from build123d import *

# Parameters (mm, degrees)
SKETCH_R        = 35
PAD_DEPTH       = 7
SKETCH002_R     = 11
POCKET_DEPTH    = 7
SKETCH003_R     = 5.25
POCKET001_DEPTH = 4
SKETCH004_R     = 2.625
POCKET002_DEPTH = 1


with BuildPart() as part:
    # Sketch → Pad (new body)
    with BuildSketch(Plane.XY):
        Circle(SKETCH_R)
    extrude(amount=PAD_DEPTH)

    # Sketch002 → Pocket (cut)
    with BuildSketch(Plane(origin=(0, 0, 0), x_dir=(1, 0, 0), z_dir=(0, 0, -1))):
        Circle(SKETCH002_R)
    extrude(amount=-POCKET_DEPTH, mode=Mode.SUBTRACT)

    # Sketch003 (on Face3 of Pocket) → Pocket001 (cut)
    with BuildSketch(Plane.XY.offset(7)):
        with Locations((20, 0)):
            Circle(SKETCH003_R)
        with Locations((-20, 0)):
            Circle(SKETCH003_R)
    extrude(amount=-POCKET001_DEPTH, mode=Mode.SUBTRACT)

    # Sketch004 (on Face7 of Pocket001) → Pocket002 (cut)
    with BuildSketch(Plane.XY.offset(3)):
        with Locations((-20, 0)):
            Circle(SKETCH004_R)
        with Locations((20, 0)):
            Circle(SKETCH004_R)
    extrude(amount=-POCKET002_DEPTH, mode=Mode.SUBTRACT)


solid = part.part
The model under review builds one solid part; all positions refer to its coordinate system, in mm. A direction names the side the tool comes from. Give positions to 0.01 mm unless a question says otherwise; leave off trailing zeros. Loops run counter-clockwise (first coordinate to the right, second up) from the corner with the lowest first, then second, coordinate; pieces in that order, holes last. Notation, with made-up numbers: (57.5, 20.5) -> (86.5, 20.5) arc R15 ccw to (86.5, 49.5) -> close; hole circle Ø11 at (-0.5, 21). An arc over 180 degrees is marked (long way). Put each result on its own line as item: value. Start each with the question number.
1. For faces 1 (the face through (14.755, 0.231, 5.028)), 2 (the face through (-8, 8, 7)), list the 3-axis set-ups (+Z, -Z, +X, -X, +Y, -Y) from which the entire face can be reached by the end or side of a thin tool; tool diameter is ignored.
2. We need section A-A on x = 0. State the section outline as (y, z) points, then the cut area to 3 significant figures.
3. We need section B-B on y = 0. State the section outline as (x, z) points (3 decimals).
4. Mouldability with a two-part tool opening along Y and no side actions: class faces 3 (the face through (-2.38, 10.74, 3.45)), 4 (the face through (-8, 8, 0)), 5 (the face through (-28, -21, 3)) as released by +Y, released by -Y, zero draft, split by the parting line, or undercut.
5. Wall thickness on probe 1 along X at (y, z) = (1.5, 5.75); probe 2 along X at (y, z) = (10, 3.25); probe 3 along Y at (x, z) = (20, 4.85): over which ranges is each line inside the solid? List them lowest first.
6. We need section C-C on z = 5. State the section outline as (x, y) points, then the cut area to 3 significant figures.
7. We need section D-D on y = 9. State the section outline as (x, z) points.
8. Clearance check with flat-ended pins moving along their axes: P1, Ø1.5, axis at x = 14.5, z = 5, coming from the +Y side; P2, Ø2.5, axis at x = 20.5, y = -1, coming from the +Z side; P3, Ø9.5, axis at x = 20, y = 0, coming from the +Z side. State where each tip first meets the part, or that it passes through.
Determined:
1. face 1: +Z
1. face 2: +Z, +X, -X, +Y, -Y
2. outline: (-35, 0) -> (-11, 0) -> (-11, 7) -> (-35, 7) -> close; (11, 0) -> (35, 0) -> (35, 7) -> (11, 7) -> close
2. area: 336 mm^2
3. outline: (-35, 0) -> (-11, 0) -> (-11, 7) -> (-14.75, 7) -> (-14.75, 3) -> (-17.375, 3) -> (-17.375, 2) -> (-22.625, 2) -> (-22.625, 3) -> (-25.25, 3) -> (-25.25, 7) -> (-35, 7) -> close; (11, 0) -> (35, 0) -> (35, 7) -> (25.25, 7) -> (25.25, 3) -> (22.625, 3) -> (22.625, 2) -> (17.375, 2) -> (17.375, 3) -> (14.75, 3) -> (14.75, 7) -> (11, 7) -> close
4. face 3: undercut
4. face 4: zero draft
4. face 5: split by the parting line
5. probe 1: -34.97 to -25.03, -14.97 to -10.9, 10.9 to 14.97, 25.03 to 34.97
5. probe 2: -33.54 to -4.58, 4.58 to 33.54
5. probe 3: -28.72 to -5.25, 5.25 to 28.72
6. outline: circle Ø70 at (0, 0); hole circle Ø10.5 at (-20, 0); hole circle Ø22 at (0, 0); hole circle Ø10.5 at (20, 0)
6. area: 3,300 mm^2
7. outline: (-33.82, 0) -> (-6.32, 0) -> (-6.32, 7) -> (-33.82, 7) -> close; (6.32, 0) -> (33.82, 0) -> (33.82, 7) -> (6.32, 7) -> close
8. P1: y = 32.19
8. P2: z = 2
8. P3: z = 3
